Here's how the part is built. I have some questions about the finished solid (model axes, mm). Round coordinates to 2 decimals unless told otherwise and drop trailing zeros. Order: outer loops, then holes, each group sorted by start corner. A loop starts at its lowest first (then second) coordinate and runs counter-clockwise, first axis right, second up.
```python
from build123d import *

# Parameters (mm, degrees)
SKETCH1_W           = 901.6
SKETCH1_H           = 101.6
BOSS_EXTRUDE1_DEPTH = 50.8
CUT_EXTRUDE1_DEPTH  = 51.8
FILLET1_R           = 5.08


with BuildPart() as part:
    # Sketch1 → Boss-Extrude1 (new body)
    with BuildSketch(Plane(origin=(0, -12.7, 0), x_dir=(-1, 0, 0), z_dir=(0, -1, 0))):
        with Locations((-2263.5, 338.5)):
            Rectangle(SKETCH1_W, SKETCH1_H)
    extrude(amount=-BOSS_EXTRUDE1_DEPTH)

    # Sketch3 → Cut-Extrude1 (cut, through all)
    with BuildSketch(Plane(origin=(0, 38.1, 0), x_dir=(1, 0, 0), z_dir=(0, 1, 0))):
        Polygon((2549.2, 287.7), (2600, 326.680210989), (2650.8, 287.7), align=None)
        Polygon((1812.7, 338.5), (1812.7, 287.7), (1863.5, 287.7), align=None)
    extrude(amount=-CUT_EXTRUDE1_DEPTH, mode=Mode.SUBTRACT)

    # Fillet1
    fillet1_edges = [part.edges().sort_by_distance(p)[0] for p in [
        (2206.35, -12.7, -287.7),
        (1812.7, -12.7, -363.9),
        (2263.5, 38.1, -389.3),
        (1812.7, 38.1, -363.9),
        (2206.35, 38.1, -287.7),
        (2574.6, -12.7, -307.190105495),
        (2625.4, -12.7, -307.190105495),
        (2625.4, 38.1, -307.190105495),
        (2574.6, 38.1, -307.190105495),
        (1838.1, -12.7, -313.1),
        (1838.1, 38.1, -313.1),
        (2714.3, 38.1, -338.5),
        (2263.5, -12.7, -389.3),
        (2682.55, -12.7, -287.7),
        (2714.3, -12.7, -338.5),
        (2682.55, 38.1, -287.7),
    ]]
    fillet(fillet1_edges, radius=FILLET1_R)


solid = part.part
```
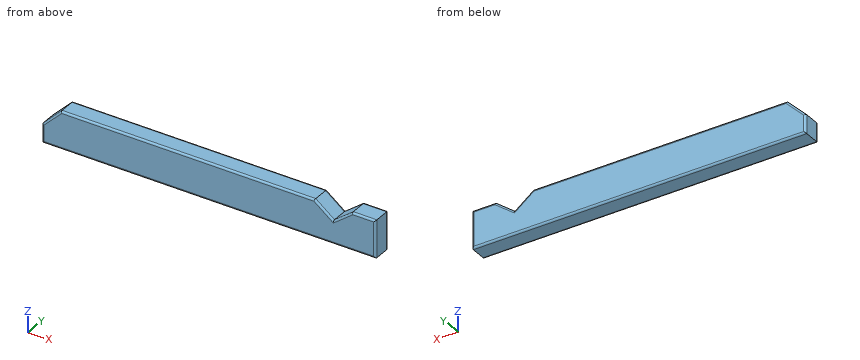
1. I'm going to push a flat-ended pin straight in: P1, Ø10, axis at y = 29, z = -300.5, coming from the -X side. Where does the tip first touch, or does it pass through?
Evaluation:
P1: stops at x = 1845.7
2. I need wall thicknesses on probe 1 along X at (y, z) = (10.5, -323.5); probe 2 along X at (y, z) = (31, -304); probe 3 along Z at (x, y) = (2587, 1.5). Which ranges of each line are inside material? Lowest first, please.
Evaluation:
probe 1: x = 1827.7 to 2595.86, 2604.14 to 2714.3
probe 2: x = 1847.2 to 2570.44, 2629.56 to 2714.3
probe 3: z = -389.3 to -316.7
3. If we section it at A-A, the plane y = 0: Write out the boundary of the cut face in (x, z), and give its area (3 significant figures).
Evaluation:
outline: (1812.7, -389.3) - (2714.3, -389.3) - (2714.3, -287.7) - (2650.8, -287.7) - (2600, -326.68) - (2549.2, -287.7) - (1863.5, -287.7) - (1812.7, -338.5) - close
area: 88,300 mm2
